Work out the finished part from the listing and answer in its coordinate system (mm). Coordinates: 2 decimals unless noted, no trailing zeros. Write each loop counter-clockwise with the first axis right and the second up, starting at its lowest first coordinate (ties: lowest second). Pieces come first, ordered by that corner, then holes. Notation, with made-up numbers: (67.25, -31) - (98.25, -31) arc R25 ccw to (98.25, -8) - close; hole circle Ø1 at (41, 64). An arc over 180 degrees is marked (long way). Answer as a JSON object with one key per item and string values. Group by question number.
Autodesk Inventor part; units mm, degrees
ref_plane "YZ Plane" through (0, 0, 0) normal (1, 0, 0) x (0, 1, 0)
ref_plane "XZ Plane" through (0, 0, 0) normal (0, 1, 0) x (-1, 0, 0)
ref_plane "XY Plane" through (0, 0, 0) normal (0, 0, 1) x (1, 0, 0)
sketch "Sketch1" plane through (0, 0, 0) normal (1, 0, 0) x (0, 1, 0)
  circle A0 centre (0, 0) radius 158.2356
  dimension "d0" = 316.4711
extrude "Extrusion1" add sketch "Sketch1" along normal blind 6.35
sketch "Sketch2" plane through (0, 0, 0) normal (-1, 0, 0) x (0, 0, 1)
  circle A0 centre (0, 145.5356) radius 3.3782
  point P0 (0, 0)
  dimension "d3" = 6.7564
  dimension "d4" = 145.5356
extrude "Extrusion2" cut sketch "Sketch2" against normal through all
sketch "Sketch3" plane through (0, 0, 0) normal (-1, 0, 0) x (0, 0, 1)
  point P0 (0, 0)
  point P1 (23.8125, 0)
  point P2 (11.9063, 20.6222)
  point P3 (-11.9062, 20.6222)
  point P4 (-23.8125, 0)
  point P5 (-11.9063, -20.6222)
  point P6 (11.9062, -20.6222)
  dimension "d7" = 23.8125
  dimension "d10" = 360
hole "Hole1" at (0, 0, 23.8125) at (0, 20.6222, 11.9063) at (0, 20.6222, -11.9062) at (0, 0, -23.8125) at (0, -20.6222, -11.9063) at (0, -20.6222, 11.9062) direction (1, 0, 0) diameter 3.048 end through all
sketch "Sketch6" plane through (0, 0, 0) normal (-1, 0, 0) x (0, 0, 1)
  arc A0 (-25.4, 28.3981) -> (25.4, 28.3981) centre (0, 0) ccw
  line L0 (-25.4, 28.3981) -> (-25.4, 156.1837)
  circle A1 centre (0, 0) radius 158.2356
  line L1 (25.4, 28.3981) -> (25.4, 156.1837)
  dimension "d29" = 25.4
  dimension "d30" = 25.4
  dimension "d31" = 76.2
extrude "Extrusion4" cut sketch "Sketch6" against normal through all contours A0 L1 A1 L0 picked at (-31.115, 112.3302)
equation "\"d0\" = camPlateDiam"
equation "\"d1\" = camPlateThickness"
equation "\"d3\" = camPostHoleDiam"
equation "\"d5\" = camPlateThickness"
equation "\"camPlateThickness\" = 6.35"
equation "\"camPostHoleDiam\" = 6.7564"
equation "\"camPostHeight\" = 25.4"
equation "\"camRadius\" = 0.5 * camDiam"
equation "\"aM6HoleDiam\" = 47.625"
equation "\"am6HoleRadius\" = 0.5 * aM6HoleDiam"
equation "\"centerHoleDiam\" = 28.575"
equation "\"camStroke\" = 152.4"
equation "\"pi\" = 79.7941"
properties part number "camPlate" material "Aluminum 6061"
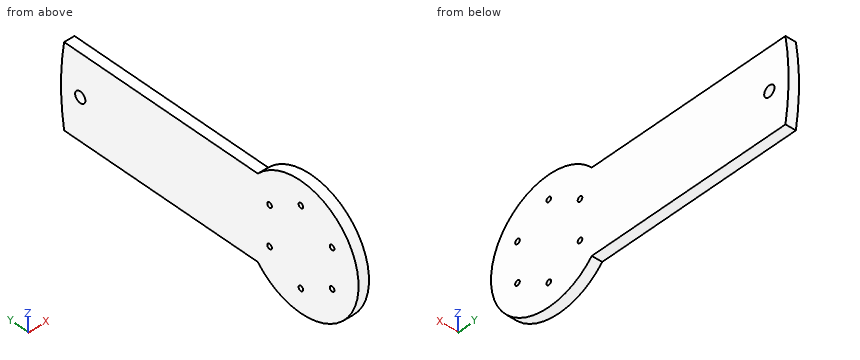
Q1. Flat-ended cylindrical pins translate along their axes: pin 1 Ø3 at (x, z) = (2, -26.5) entering from +Y; pin 2 Ø1.5 at (x, z) = (5.5, -12.5) entering from -Y; pin 3 Ø2 at (x, y) = (3, 11) entering from +Z. Find the tip coordinate at first contact, or state that the pin passes through.
Q2. Section A-A on z = 0 is taken. Determine the outline of the cut face in (x, y).
Q3. Section B-B on x = 5.25 is taken. Determine the outline of the cut face in (y, z).
Q4. Section D-D on z = -16.5 is taken. Determine the outline of the cut face in (x, y).
Q5. Section C-C on y = 98 is taken. Determine the outline of the cut face in (x, z), plus the area to 3 significant figures.
Q6. Consider L1, parallel to Y at x = 1, z = -2; L2, parallel to Y at x = 4, z = -25; L3, parallel to Z at x = 2, y = 108. Determine where each line is inside the solid, lowest interval first. Write a range as from..to.
Numbers:
{
 "1": {"pin 1": "stops at y = 156.25", "pin 2": "stops at y = -36.24", "pin 3": "stops at z = 36.76"},
 "2": {"outline": "(0, -38.1) - (6.35, -38.1) - (6.35, 142.16) - (0, 142.16) - close; (0, 148.91) - (6.35, 148.91) - (6.35, 158.24) - (0, 158.24) - close"},
 "3": {"outline": "(28.4, -25.4) - (156.18, -25.4) arc R158.24 ccw to (156.18, 25.4) - (28.4, 25.4) arc R38.1 ccw (long way) to start; hole circle Ø3.05 at (-20.62, -11.91); hole circle Ø3.05 at (-20.62, 11.91); hole circle Ø3.05 at (0, -23.81); hole circle Ø3.05 at (0, 23.81); hole circle Ø3.05 at (20.62, -11.91); hole circle Ø3.05 at (20.62, 11.91); hole circle Ø6.76 at (145.54, 0)"},
 "4": {"outline": "(0, -34.34) - (6.35, -34.34) - (6.35, 157.37) - (0, 157.37) - close"},
 "5": {"outline": "(0, -25.4) - (6.35, -25.4) - (6.35, 25.4) - (0, 25.4) - close", "area": "323 mm²"},
 "6": {"L1": "y = -38.05..142.81, 148.26..158.22", "L2": "y = -28.75..-0.96, 0.96..156.25", "L3": "z = -25.4..25.4"}
}
